```python
from build123d import *

# Parameters (mm, degrees)
SKETCH1_W           = 25.146
SKETCH1_H           = 177.8
BOSS_EXTRUDE1_DEPTH = 5.08
BOSS_EXTRUDE3_DEPTH = 10.16
SKETCH4_W           = 25.146
SKETCH4_H           = 25.485835905
CUT_EXTRUDE1_DEPTH  = 2.54
SKETCH5_R           = 3
CUT_EXTRUDE2_DEPTH  = 133.167293803
SKETCH6_R           = 6
SKETCH6_R_2         = 3
CUT_EXTRUDE3_DEPTH  = 16.51
CUT_EXTRUDE4_DEPTH  = 133.167293803


with BuildPart() as part:
    # Sketch1 → Boss-Extrude1 (new body)
    with BuildSketch(Plane(origin=(0, 0, 0), x_dir=(1, 0, 0), z_dir=(0, 1, 0))):
        with Locations((-33.02, -34.737560241)):
            Rectangle(SKETCH1_W, SKETCH1_H)
    extrude(amount=BOSS_EXTRUDE1_DEPTH)

    # Sketch3 → Boss-Extrude3 (add)
    with BuildSketch(Plane(origin=(0, 5.08, 0), x_dir=(1, 0, 0), z_dir=(0, 1, 0))):
        Polygon((-38.481, -123.637560241), (-20.447, -123.637560241), (-20.447, -118.557560241), (-33.401, -118.557560241), (-33.401, 18.602439759), (-20.447, 18.602439759), (-20.447, 19.76859762), (-38.481, 19.76859762), align=None)
    extrude(amount=BOSS_EXTRUDE3_DEPTH)

    # Sketch4 → Cut-Extrude1 (cut)
    with BuildSketch(Plane(origin=(0, 5.08, 0), x_dir=(1, 0, 0), z_dir=(0, 1, 0))):
        with Locations((-33.02, 41.419521807)):
            Rectangle(SKETCH4_W, SKETCH4_H)
    extrude(amount=-CUT_EXTRUDE1_DEPTH, mode=Mode.SUBTRACT)

    # Sketch5 → Cut-Extrude2 (cut, through all)
    with BuildSketch(Plane(origin=(0, 5.08, 0), x_dir=(1, 0, 0), z_dir=(0, 1, 0))):
        with Locations(Location((-33.02, 24.222600737, 0), (0, 0, 270))):
            Circle(SKETCH5_R)
    extrude(amount=-CUT_EXTRUDE2_DEPTH, mode=Mode.SUBTRACT)

    # Sketch6 → Cut-Extrude3 (cut)
    with BuildSketch(Plane(origin=(0, 5.08, 0), x_dir=(1, 0, 0), z_dir=(0, 1, 0))):
        with Locations((-42.037, -85.537560241)):
            Circle(SKETCH6_R)
        with Locations((-42.037, -85.537560241)):
            Circle(SKETCH6_R_2, mode=Mode.SUBTRACT)
    extrude(amount=CUT_EXTRUDE3_DEPTH, mode=Mode.SUBTRACT)

    # Sketch6<3> → Cut-Extrude4 (cut, through all)
    with BuildSketch(Plane(origin=(0, 5.08, 0), x_dir=(1, 0, 0), z_dir=(0, 1, 0))):
        with BuildLine():
            ThreePointArc((-42.037, -82.537560241), (-45.037, -85.537560241), (-42.037, -88.537560241))
            Line((-42.037, -88.537560241), (-42.037, -82.537560241))
        make_face()
        with BuildLine():
            Line((-42.037, -82.537560241), (-42.037, -88.537560241))
            ThreePointArc((-42.037, -88.537560241), (-39.915679656, -87.658880585), (-39.037, -85.537560241))
            ThreePointArc((-39.037, -85.537560241), (-39.915679656, -83.416239897), (-42.037, -82.537560241))
        make_face()
    extrude(amount=-CUT_EXTRUDE4_DEPTH, mode=Mode.SUBTRACT)


solid = part.part
```
Here's how the part is built. I have some questions about the finished solid (model axes, mm). A direction names the side the tool comes from. Round coordinates to 2 decimals unless told otherwise and drop trailing zeros. Order: outer loops, then holes, each group sorted by start corner. A loop starts at its lowest first (then second) coordinate and runs counter-clockwise, first axis right, second up. Notation, with made-up numbers: (46, -38) -> (56, -38) arc R24 cw to (56, -28) -> close; hole circle Ø6 at (17.25, 13.25). An arc over 180 degrees is marked (long way). Use a Markdown table: item, result. Add a question column.
(1) I need wall thicknesses on line 1 along Z through (x, y) = (-33, 10); line 2 along Y through (x, z) = (-34, -37); line 3 along X through (y, z) = (13.5, 44.5). Which ranges of each line are inside material? Lowest first, please.
(2) For pin 1 Ø9.5 at (x, z) = (-33.02, -24.22) entering from +Y; pin 2 Ø3 at (x, y) = (-25.5, 11) entering from -Z; pin 3 Ø5 at (y, z) = (9.5, -2.5) entering from +X; pin 4 Ø3 at (y, z) = (11.5, 25) entering from -X, each with a flat end and sliding along its axis, tell me the tip position at first contact or that it passes through.
(3) For faces 4 (the face through (-33, 2.54, -42)), 5 (the face through (-36.038, 10.089, 85.616)), 6 (the face through (-27, 5.08, 49)), 7 (the face through (-38.481, 10, 107)), which set-ups out of +Z, -Z, +X, -X, +Y, -Y let a thin tool reach every point of the face, with its end or its side?
(4) Suppose I cut it at C-C, the plane z = 40.5. Please give me the cut outline in (x, y).
(5) If we mould it in two halves opening along X, with no side actions, what happens to faces 1 (the face through (-33, 0, 33)), 2 (the face through (-33.401, 10, 51)), 3 (the face through (-30.046, 2.576, -24.613))? For each: released by +X, released by -X, zero draft, split by the parting line, or undercut.
(6) Suppose I cut it at A-A, the plane x = -43.5. Please give me the cut outline in (y, z), and give its area (3 significant figures).
(7) Suppose I cut it at B-B, the plane y = 8.5. Please give me the cut outline in (x, z).
Verdict:
| question | item | result |
|---|---|---|
| 1 | line 1 | -19.77 to -18.6, 118.56 to 123.64 |
| 1 | line 2 | 0 to 2.54 |
| 1 | line 3 | -38.48 to -33.4 |
| 2 | pin 1 | y = 15.24 |
| 2 | pin 2 | z = -19.77 |
| 2 | pin 3 | x = -33.4 |
| 2 | pin 4 | x = -38.48 |
| 3 | face 4 | -Z, +X, -X, +Y |
| 3 | face 5 | -X, +Y |
| 3 | face 6 | +X, +Y |
| 3 | face 7 | +Z, -Z, -X, +Y |
| 4 | outline | (-45.59, 0) -> (-20.45, 0) -> (-20.45, 5.08) -> (-33.4, 5.08) -> (-33.4, 15.24) -> (-38.48, 15.24) -> (-38.48, 5.08) -> (-45.59, 5.08) -> close |
| 5 | face 1 | zero draft |
| 5 | face 2 | released by +X |
| 5 | face 3 | undercut |
| 6 | outline | (0, -54.16) -> (2.54, -54.16) -> (2.54, -28.68) -> (5.08, -28.68) -> (5.08, 82.92) -> (0, 82.92) -> close; (0, 88.16) -> (5.08, 88.16) -> (5.08, 123.64) -> (0, 123.64) -> close |
| 6 | area | 812 mm2 |
| 7 | outline | (-38.48, -19.77) -> (-20.45, -19.77) -> (-20.45, -18.6) -> (-33.4, -18.6) -> (-33.4, 118.56) -> (-20.45, 118.56) -> (-20.45, 123.64) -> (-38.48, 123.64) -> (-38.48, 90.37) arc R6 cw to (-38.48, 80.7) -> close |
